Input: part model. Units: mm. Frame: model coordinates. Face numbers are marked on the shaded views. Coordinates: 2 decimals unless noted, no trailing zeros. Order: outer loops, then holes, each group sorted by start corner. A loop starts at its lowest first (then second) coordinate and runs counter-clockwise, first axis right, second up. Notation, with made-up numbers: (-14, 19) - (14, 19) arc R23 cw to (14, 46) - close; hole circle Ø11 at (34, -33.5). An arc over 180 degrees is marked (long way). One line per question, with ' | ' between items. Start each with the question number.
```python
from build123d import *

# Parameters (mm, degrees)
F0_R     = 7.5
F1_DEPTH = 25


with BuildPart() as f1:
    # F0 (on Front) → F1 (new body)
    with BuildSketch(Plane.XZ):
        with BuildLine():
            ThreePointArc((-9.511187, -11.599023), (6.416081, -13.558536), (15, 0))
            ThreePointArc((15, 0), (0, 15), (-15, 0))
            ThreePointArc((-15, 0), (-13.558536, -6.416081), (-9.511187, -11.599023))
        make_face()
        Circle(F0_R, mode=Mode.SUBTRACT)
        with BuildLine():
            ThreePointArc((-9.511187, -11.599023), (-13.558536, -6.416081), (-15, 0))
            ThreePointArc((-15, 0), (-124.111916, -62.094191), (-245.884248, -92.632656))
            ThreePointArc((-245.884248, -92.632656), (-242.019707, -97.753195), (-240.647886, -104.019989))
            ThreePointArc((-240.647886, -104.019989), (-133.191596, -112.174328), (-55.899361, -187.26932))
            ThreePointArc((-55.899361, -187.26932), (-49.492549, -182.278121), (-41.423323, -181.357856))
            ThreePointArc((-41.423323, -181.357856), (-59.069676, -90.161684), (-9.511187, -11.599023))
        make_face()
        with BuildLine():
            ThreePointArc((-240.647886, -104.019989), (-242.019707, -97.753195), (-245.884248, -92.632656))
            ThreePointArc((-245.884248, -92.632656), (-269.276066, -110.286784), (-240.647886, -104.019989))
        make_face()
        with Locations((-255.647886, -104.019989)):
            Circle(F0_R, mode=Mode.SUBTRACT)
        with BuildLine():
            ThreePointArc((-28.821729, -196.16487), (-32.398592, -186.443144), (-41.423323, -181.357856))
            ThreePointArc((-41.423323, -181.357856), (-49.492549, -182.278121), (-55.899361, -187.26932))
            ThreePointArc((-55.899361, -187.26932), (-48.50337, -210.415562), (-28.821729, -196.16487))
        make_face()
        with Locations((-43.821729, -196.16487)):
            Circle(F0_R, mode=Mode.SUBTRACT)
    extrude(amount=F1_DEPTH)


solid = f1.part
```
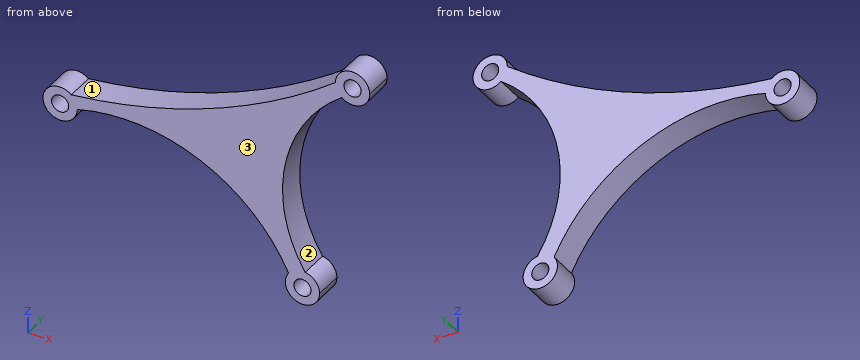
(1) Section A-A (x = 0). Output: boundary loops of the cut face in (y, z).
(2) Pin query (flat end, axial travel): pin 1 (12 mm diameter, centred on x = -43.82, z = -196.16, fed in from -Y); pin 2 (3 mm diameter, centred on x = -31, y = -6, fed in from -Z); pin 3 (12 mm diameter, centred on x = -195.5, y = -5.5, fed in from +Z); pin 4 (12 mm diameter, centred on y = -15, z = -102, fed in from +X). Return the tip coordinate at first contact, or that it passes through.
(3) Material intervals for line 1 along Z through (x, y) = (-256, -5.5); line 2 along Z through (x, y) = (0, -19.5); line 3 along X through (y, z) = (-23, -110), sorted ascending. Write a range as from..to.
(4) Section C-C (z = -50.5). Output: boundary loops of the cut face in (x, y).
(5) Draft query along Z for the marked faces 1, 2 and 3. Return one class per face: +Z half, -Z half, draft (parallel to the pull), parting line (faces both ways), or undercut.
(6) Section D-D (x = -99.5). Output: boundary loops of the cut face in (y, z).
(7) Section B-B (y = -5). Output: boundary loops of the cut face in (x, z).
Worked answers:
1) outline: (-25, -15) - (0, -15) - (0, -7.5) - (-25, -7.5) - close; (-25, 7.5) - (0, 7.5) - (0, 15) - (-25, 15) - close
2) pin 1: passes through | pin 2: stops at z = -206 | pin 3: stops at z = -82.86 | pin 4: stops at x = -60.03
3) line 1: z = -119.02..-111.51, -96.53..-89.02 | line 2: z = -15..-7.5, 7.5..15 | line 3: x = -269.4..-260.17, -251.12..-241.89, -138.25..-61.19
4) outline: (-97.63, -25) - (-44.4, -25) - (-44.4, 0) - (-97.63, 0) - close
5) face 1: +Z half | face 2: undercut | face 3: draft
6) outline: (-25, -132.76) - (0, -132.76) - (0, -51.38) - (-25, -51.38) - close
7) outline: (-245.88, -92.63) arc R15 ccw (long way) to (-240.65, -104.02) arc R158.17 cw to (-55.9, -187.27) arc R15 ccw (long way) to (-41.42, -181.36) arc R126.18 cw to (-9.51, -11.6) arc R15 ccw (long way) to (-15, 0) arc R463.55 cw to start; hole circle Ø15 at (-255.65, -104.02); hole circle Ø15 at (-43.82, -196.16); hole circle Ø15 at (0, 0)
